```python
from build123d import *

# Parameters (mm, degrees)
SKETCH_1_R        = 16.5
SKETCH_1_R_2      = 7.5
EXTRUDE_1_DEPTH   = 8
HOLE_WIZARD_M31_D = 3.4
M4X0_71_REACH     = 39.752
M4X0_71_BORE_R    = 1.65
M4X0_72_REACH     = 39.752
M4X0_72_BORE_R    = 1.65


with BuildPart() as part:
    # Эскиз1 → Бобышка-Вытянуть1 (new body)
    with BuildSketch(Plane.XY):
        Circle(SKETCH_1_R)
        Circle(SKETCH_1_R_2, mode=Mode.SUBTRACT)
    extrude(amount=EXTRUDE_1_DEPTH)

    # Отверстие с зазором M31 (through all)
    with Locations(Plane.XY.offset(8)):
        with Locations((-6.25, 10.825317547), (12.5, 0), (-6.25, -10.825317547)):
            Hole(HOLE_WIZARD_M31_D / 2)

    # Отверстие обработанное метчиком M4x0.71 bore → Отверстие обработанное метчиком M4x0.71 (cut, up to next)
    with BuildSketch(Plane.ZY.offset(16.5), mode=Mode.PRIVATE) as m4x0_71_sk1:
        with Locations((4, 0)):
            Circle(M4X0_71_BORE_R)
    m4x0_71_tool1 = extrude(m4x0_71_sk1.sketch, amount=-M4X0_71_REACH, mode=Mode.PRIVATE) & part.part
    add(m4x0_71_tool1.solids().sort_by_distance((-16.5, 0, 4))[0], mode=Mode.SUBTRACT)

    # Отверстие обработанное метчиком M4x0.72 bore → Отверстие обработанное метчиком M4x0.72 (cut, up to next)
    with BuildSketch(Plane.ZX.offset(16.5), mode=Mode.PRIVATE) as m4x0_72_sk1:
        with Locations((4, 0)):
            Circle(M4X0_72_BORE_R)
    m4x0_72_tool1 = extrude(m4x0_72_sk1.sketch, amount=-M4X0_72_REACH, mode=Mode.PRIVATE) & part.part
    add(m4x0_72_tool1.solids().sort_by_distance((0, 16.5, 4))[0], mode=Mode.SUBTRACT)


solid = part.part
```
The model under review builds one solid part; all positions refer to its coordinate system, in mm. A direction names the side the tool comes from. Coordinates: 2 decimals unless noted, no trailing zeros. Write each loop counter-clockwise with the first axis right and the second up, starting at its lowest first coordinate (ties: lowest second). Pieces come first, ordered by that corner, then holes.
1) We need section D-D on x = 12. State the section outline as (y, z) points, then the cut area to 3 significant figures.
2) We need section A-A on z = 4. State the section outline as (x, y) points.
3) We need section B-B on x = 0. State the section outline as (y, z) points, then the cut area to 3 significant figures.
4) The part is to be moulded in two halves that separate along Y. For faces 1 (the face through (7.1, -3.4, 0)), 2 (the face through (-11.97, 0.07, 2.35)), 3 (the face through (15.738, 4.956, 3.944)), say which applies: pulls with the +Y half, pulls with the -Y half, needs draft (parallel to the pull), parting line crosses it, or undercut.
5) To check wall thickness, follow probe 1 along Y at (x, z) = (-6.25, 5); probe 2 along Y at (x, z) = (-6, 3.25); probe 3 along Y at (x, z) = (0, 3.5). State the ranges of each line that lie inside material, in increasing order.
6) Machinability: for faces 4 (the face through (-4.55, 10.9, 3.94)), 5 (the face through (0.07, 11.97, 2.35)), which of the approach directions +Z, -Z, +X, -X, +Y, -Y give a long, thin tool a straight path to every point of the face, cutting with its end or side? Answer none if there is none.
7) We need section C-C on y = 0. State the section outline as (x, z) points, then the cut area to 3 significant figures.
8) Clearance check with flat-ended pins moving along their axes: pin 1 Ø4 at (y, z) = (6, 3.5) entering from +X; pin 2 Ø1.5 at (x, z) = (-2.5, 5.5) entering from +Y; pin 3 Ø1 at (x, z) = (5, 6) entering from -Y. State where each tip first meets the part, or that it passes through.
Answer list:
1. outline: (-11.32, 0) - (-1.62, 0) - (-1.62, 8) - (-11.32, 8) - close; (1.62, 0) - (11.32, 0) - (11.32, 8) - (1.62, 8) - close
1. area: 155 mm2
2. outline: (-16.42, -1.65) arc R16.5 ccw (long way) to (1.65, 16.42) - (1.65, 7.32) arc R7.5 cw (long way) to (-7.32, -1.65) - close; (-16.42, 1.65) - (-7.32, 1.65) arc R7.5 cw to (-1.65, 7.32) - (-1.65, 16.42) arc R16.5 ccw to start; hole circle Ø3.4 at (-6.25, -10.83); hole circle Ø3.4 at (-6.25, 10.83); hole circle Ø3.4 at (12.5, 0)
3. outline: (-16.5, 0) - (-7.5, 0) - (-7.5, 8) - (-16.5, 8) - close; (7.5, 0) - (16.5, 0) - (16.5, 2.35) - (7.5, 2.35) - close; (7.5, 5.65) - (16.5, 5.65) - (16.5, 8) - (7.5, 8) - close
3. area: 114 mm2
4. face 1: needs draft
4. face 2: undercut
4. face 3: parting line crosses it
5. probe 1: y = -15.27 to -12.53, -9.13 to -4.15, 4.15 to 9.13, 12.53 to 15.27
5. probe 2: y = -15.37 to -12.51, -9.14 to -4.5, 4.5 to 9.14, 12.51 to 15.37
5. probe 3: y = -16.5 to -7.5
6. face 4: +Z, -Z
6. face 5: +Y
7. outline: (-16.5, 0) - (-7.5, 0) - (-7.5, 2.35) - (-16.5, 2.35) - close; (-16.5, 5.65) - (-7.5, 5.65) - (-7.5, 8) - (-16.5, 8) - close; (7.5, 0) - (10.8, 0) - (10.8, 8) - (7.5, 8) - close; (14.2, 0) - (16.5, 0) - (16.5, 8) - (14.2, 8) - close
7. area: 87.1 mm2
8. pin 1: stops at x = 16.01
8. pin 2: stops at y = 16.41
8. pin 3: stops at y = -15.87
